```python
from build123d import *

# Parameters (mm, degrees)
SKETCH1_W               = 100
SKETCH1_H               = 60
SKETCH1_R               = 1.75
BOSS_EXTRUDE1_DEPTH     = 2.5
SKETCH2_W               = 15
SKETCH2_H               = 15
BOSS_EXTRUDE2_DEPTH     = 9
MIRROR2_COPY_1_SKETCH_W = 15
MIRROR2_COPY_1_SKETCH_H = 15
MIRROR2_COPY_1_DEPTH    = 9
FILLET1_R               = 2.5
FILLET2_R               = 2.5
CHAMFER1_SIZE           = 2.5


with BuildPart() as part:
    # Sketch1 → Boss-Extrude1 (new body)
    with BuildSketch(Plane.XY):
        with Locations((-12.5, 0)):
            Rectangle(SKETCH1_W, SKETCH1_H)
        Polygon((-34, -26.5), (-34, 26.5), (-22.75, 26.5), (-22.75, 19), (-16.5, 19), (-16.5, 26.5), (34, 26.5), (34, 12.25), (26.5, 12.25), (26.5, 4.75), (34, 4.75), (34, -15.75), (26.5, -15.75), (26.5, -23.25), (34, -23.25), (34, -26.5), (-16.55, -26.5), (-16.55, -19), (-24.05, -19), (-24.05, -26.5), align=None, mode=Mode.SUBTRACT)
        with Locations((-19, 24)):
            Circle(SKETCH1_R, mode=Mode.SUBTRACT)
        with Locations((-20.3, -24)):
            Circle(SKETCH1_R, mode=Mode.SUBTRACT)
        with Locations((31.5, 8.5)):
            Circle(SKETCH1_R, mode=Mode.SUBTRACT)
        with Locations((31.5, -19.5)):
            Circle(SKETCH1_R, mode=Mode.SUBTRACT)
    extrude(amount=BOSS_EXTRUDE1_DEPTH)

    # Sketch2 → Boss-Extrude2 (add)
    with BuildSketch(Plane.XY.offset(2.5)):
        with Locations((-70, 15)):
            Rectangle(SKETCH2_W, SKETCH2_H)
    boss_extrude2 = extrude(amount=-BOSS_EXTRUDE2_DEPTH)

    # Sketch3 → Cut-Revolve1 (revolve, cut)
    with BuildSketch(Plane.ZY.offset(70), mode=Mode.PRIVATE) as cut_revolve1_sk:
        Polygon((2.5, 15), (-6.5, 15), (-6.5, 12.8), (-0.5, 12.8), (2.5, 10.192139787), align=None)
    cut_revolve1 = revolve(cut_revolve1_sk.sketch.rotate(Axis((-70, 15, 2.5), (0, 0, -1)), 270), axis=Axis((-70, 15, 2.5), (0, 0, -1)), mode=Mode.SUBTRACT)

    # Mirror1: Boss-Extrude2, Cut-Revolve1 across plane
    add(boss_extrude2.mirror(Plane.ZX))
    add(cut_revolve1.mirror(Plane.ZX), mode=Mode.SUBTRACT)

    # Mirror2: Boss-Extrude2, Cut-Revolve1 across plane
    add(boss_extrude2.mirror(Plane.ZY.offset(12.5)))
    add(cut_revolve1.mirror(Plane.ZY.offset(12.5)), mode=Mode.SUBTRACT)

    # Mirror2 copy 1 sketch → Mirror2 copy 1 (add)
    with BuildSketch(Plane(origin=(-25, 0, 2.5), x_dir=(-1, 0, 0), z_dir=(0, 0, 1))):
        with Locations((-70, 15)):
            Rectangle(MIRROR2_COPY_1_SKETCH_W, MIRROR2_COPY_1_SKETCH_H)
    extrude(amount=-MIRROR2_COPY_1_DEPTH)

    # Mirror2 copy 2 sketch → Mirror2 copy 2 (revolve, cut)
    with BuildSketch(Plane(origin=(45, 0, 0), x_dir=(0, 0, 1), z_dir=(1, 0, 0))):
        Polygon((2.5, 15), (-6.5, 15), (-6.5, 12.8), (-0.5, 12.8), (2.5, 10.192139787), align=None)
    revolve(axis=Axis((45, -15, 2.5), (0, 0, -1)), mode=Mode.SUBTRACT)

    # Fillet1
    fillet1_edges = [part.edges().sort_by_distance(p)[0] for p in [
        (-24.05, -26.5, 1.25),
        (-24.05, -19, 1.25),
        (-16.55, -26.5, 1.25),
        (34, -23.25, 1.25),
        (34, -15.75, 1.25),
        (34, 4.75, 1.25),
        (34, 12.25, 1.25),
        (-16.5, 26.5, 1.25),
        (-22.75, 26.5, 1.25),
    ]]
    fillet(fillet1_edges, radius=FILLET1_R)

    # Fillet2
    fillet2_edges = [part.edges().sort_by_distance(p)[0] for p in [
        (37.5, -30, 1.25),
        (-62.5, -30, 1.25),
        (-62.5, 30, 1.25),
        (37.5, 30, 1.25),
    ]]
    fillet(fillet2_edges, radius=FILLET2_R)

    # Chamfer1
    chamfer1_edges = [part.edges().sort_by_distance(p)[0] for p in [
        (-62.5, -15, 0),
        (-77.5, -22.5, -2),
        (-77.5, -7.5, -2),
        (37.5, -15, 0),
        (52.5, -7.5, -2),
        (52.5, -22.5, -2),
        (37.5, 15, 0),
        (52.5, 22.5, -2),
        (52.5, 7.5, -2),
        (-62.5, 15, 0),
        (-77.5, 7.5, -2),
        (-77.5, 22.5, -2),
    ]]
    chamfer(chamfer1_edges, length=CHAMFER1_SIZE)


solid = part.part
```
Can you work these out from the model? Positions are in its coordinate system, mm. A direction names the side the tool comes from. Coordinates: 2 decimals unless noted, no trailing zeros. Loops run counter-clockwise (first coordinate to the right, second up) from the corner with the lowest first, then second, coordinate; pieces in that order, holes last. Notation, with made-up numbers: (-21.5, 56.5) -> (26.5, 56.5) arc R13 cw to (26.5, 60.5) -> close; hole circle Ø2 at (-10.5, 17.25). An arc over 180 degrees is marked (long way). Put each result on its own line as item: value. Start each with the question number.
Q1. For faces 1 (the face through (-76.3, 8.8, -1.9)), 2 (the face through (37.5, 15, -4)), 3 (the face through (33.248, -15.037, 1.268)), which set-ups out of +Z, -Z, +X, -X, +Y, -Y let a thin tool reach every point of the face, with its end or its side?
Q2. I want a section at D-D (x = 45). Write out the boundary of the cut face in (y, z).
Q3. I'm going to push flat-ended pins straight in: P1, Ø5, axis at y = 0, z = -1, coming from the -X side; P2, Ø6, axis at x = 24.5, y = -18.5, coming from the -Z side; P3, Ø4.5, axis at x = 42.5, z = -4, coming from the -Y side; P4, Ø3.5, axis at x = -70, y = 15, coming from the -Z side. Where does each tip first touch, or does it pass through?
Q4. I want a section at C-C (y = -5). Write out the boundary of the cut face in (x, z).
Q5. If I drill on line 1 (Y direction, x = 31.5, z = 0.75); line 2 (X direction, y = 15, z = -2.55); line 3 (Y direction, x = 39, z = -4.25), over which ranges is the centre line in solid material (lowest first)? Write a range as [from, to].
Q6. Thinking about a two-plate mould opening in X: for faces 4 (the face through (36, 15, -1)), 5 (the face through (43, -22.5, -2)), 6 (the face through (37.5, 0, 1)), 7 (the face through (-62.5, 0, 1)), which applies, pulls with the +X half, pulls with the -X half, needs draft (parallel to the pull), parting line crosses it, or undercut?
Q7. I want a section at A-A (z = -5.25). Write out the boundary of the cut face in (x, y).
Q8. I want a section at B-B (x = 25). Write out the boundary of the cut face in (y, z), plus the area to 3 significant figures.
Taken from the geometry:
1. face 1: +Z, -Z, -X
1. face 2: -Z, +Y, -Y
1. face 3: +Z, -Z
2. outline: (-22.5, -6.5) -> (-17.2, -6.5) -> (-17.2, -0.5) -> (-19.81, 2.5) -> (-22.5, 2.5) -> close; (-12.8, -6.5) -> (-7.5, -6.5) -> (-7.5, 2.5) -> (-10.19, 2.5) -> (-12.8, -0.5) -> close; (7.5, -6.5) -> (12.8, -6.5) -> (12.8, -0.5) -> (10.19, 2.5) -> (7.5, 2.5) -> close; (17.2, -6.5) -> (22.5, -6.5) -> (22.5, 2.5) -> (19.81, 2.5) -> (17.2, -0.5) -> close
3. P1: stops at x = -62.5
3. P2: stops at z = 0
3. P3: stops at y = -22.5
3. P4: passes through
4. outline: (-62.5, 0) -> (-34, 0) -> (-34, 2.5) -> (-62.5, 2.5) -> close; (34, 0) -> (37.5, 0) -> (37.5, 2.5) -> (34, 2.5) -> close
5. line 1: y = [-30, -26.5], [-23.25, -21.25], [-17.75, -15.75], [4.75, 6.75], [10.25, 12.25], [26.5, 30]
5. line 2: x = [-77.5, -72.2], [-67.8, -62.5], [37.5, 42.8], [47.2, 52.5]
5. line 3: y = [-22.5, -7.5], [7.5, 22.5]
6. face 4: undercut
6. face 5: needs draft
6. face 6: pulls with the +X half
6. face 7: pulls with the -X half
7. outline: (-77.5, -20) -> (-75, -22.5) -> (-62.5, -22.5) -> (-62.5, -7.5) -> (-75, -7.5) -> (-77.5, -10) -> close; (-77.5, 10) -> (-75, 7.5) -> (-62.5, 7.5) -> (-62.5, 22.5) -> (-75, 22.5) -> (-77.5, 20) -> close; (37.5, -22.5) -> (50, -22.5) -> (52.5, -20) -> (52.5, -10) -> (50, -7.5) -> (37.5, -7.5) -> close; (37.5, 7.5) -> (50, 7.5) -> (52.5, 10) -> (52.5, 20) -> (50, 22.5) -> (37.5, 22.5) -> close; hole circle Ø4.4 at (-70, -15); hole circle Ø4.4 at (-70, 15); hole circle Ø4.4 at (45, -15); hole circle Ø4.4 at (45, 15)
8. outline: (-30, 0) -> (-26.5, 0) -> (-26.5, 2.5) -> (-30, 2.5) -> close; (26.5, 0) -> (30, 0) -> (30, 2.5) -> (26.5, 2.5) -> close
8. area: 17.5 mm2
